CAD build for the part. Positions are in the model's coordinates, mm. A direction names the side the tool comes from. Give positions to 0.01 mm unless a question says otherwise; leave off trailing zeros. Loops run counter-clockwise (first coordinate to the right, second up) from the corner with the lowest first, then second, coordinate; pieces in that order, holes last.
Item 1: Saw through at D-D on y = 0.5. Give the cut face in (x, z).
Item 2: Saw through at B-B on z = 2. Give the cut face in (x, y), plus the area to 3 significant figures.
Item 3: Which spindle directions (+Z, -Z, +X, -X, +Y, -Y) get a long thin tool onto all of the face, cutting with end or side? Do faces 4 (the flat face through (12, -9.083, 5)), 5 (the flat face through (-12.679, -7, 2)), 6 (the flat face through (-13.1, -5, 10)), 7 (the flat face through (-12.679, -7, 17)), 8 (the flat face through (-9, -6, 10)). Say none if no direction does.
Item 4: Saw through at C-C on x = 23.5. Give the cut face in (y, z), plus the area to 3 significant figures.
Item 5: Drop flat-ended pins along their axis: P1, Ø2.5, axis at y = -4.5, z = 6.5, coming from the -X side; P2, Ø12, axis at x = -28.5, z = 15.5, coming from the +Y side; P3, Ø1.5, axis at y = 5.5, z = 2, coming from the +X side. Give the stop position or say it passes through.
Item 6: Probe probe 1 along Y at (x, z) = (-14, 11); probe 2 along Y at (x, z) = (-4, 19); probe 3 along Y at (x, z) = (3, 10.25). List the from-to ranges inside material, lowest first.
Item 7: Mould opens along Y. For faces 1 (the flat face through (20, 1.35, 10.14)), 2 (the flat face through (-10.1, 7, 10)), 3 (the flat face through (-26, -11.5, 10)) say: released by +Y, released by -Y, zero draft, split by the parting line, or undercut.
Item 8: Saw through at A-A on y = -4.75. Give the cut face in (x, z), plus the area to 3 significant figures.
from build123d import *

# Parameters (mm, degrees)
EXTRUDE_1_DEPTH          = 20
CUT_EXTRUDE_1_DEPTH      = 49.817301935
CUT_EXTRUDE_1_DEPTH_BACK = 49.817301935
CUT_EXTRUDE_2_DEPTH      = 50.88447801
CUT_EXTRUDE_2_DEPTH_BACK = 50.88447801
SKETCH_3_W               = 26.81134726
SKETCH_3_H               = 5
CUT_EXTRUDE_3_DEPTH      = 50.88447801
CUT_EXTRUDE_3_DEPTH_BACK = 50.88447801
CUT_EXTRUDE_4_DEPTH      = 50.88447801
CUT_EXTRUDE_4_DEPTH_BACK = 50.88447801
SKETCH_5_R               = 1.55


with BuildPart() as part:
    # 草图1 → 凸台-拉伸1 (new body)
    with BuildSketch(Plane.XY):
        Polygon((-13.100304314, 11.5), (39.490013248, 11.5), (39.490013248, -9.083192704), (1.044300056, -9.083192704), (-7.416317872, -10.795276425), (-10.024002967, -11.323036202), (-12.678665988, -11.5), (-39.490013248, -11.5), (-39.490013248, -7.536083067), (-13.100304314, -7.5), (-13.100304314, -3), (-10.100304314, -3), (-10.100304314, -6), (-7.100304314, -6), (-7.100304314, -2.65), (-3.000304314, -2.65), (-3.000304314, 5.15), (-7.100304314, 5.15), (-7.100304314, 8.5), (-10.100304314, 8.5), (-10.100304314, 5.5), (-13.100304314, 5.5), align=None)
    extrude(amount=EXTRUDE_1_DEPTH)

    # 草图2 → 切除-拉伸1 (cut, two sides: drawn at the far end of the back side and taken through both)
    with BuildSketch(Plane.XZ.offset(9.083192704).offset(-CUT_EXTRUDE_1_DEPTH_BACK)):
        Polygon((1.044300056, 20), (39.490013248, 0), (39.490013248, 20), align=None)
    extrude(amount=CUT_EXTRUDE_1_DEPTH + CUT_EXTRUDE_1_DEPTH_BACK, mode=Mode.SUBTRACT)

    # 草图3 → 切除-拉伸2 (cut, two sides: drawn at the far end of the back side and taken through both)
    with BuildSketch(Plane.XZ.offset(11.5).offset(-CUT_EXTRUDE_2_DEPTH_BACK)):
        with Locations((-26.084339618, 17.5)):
            Rectangle(SKETCH_3_W, SKETCH_3_H)
        with Locations((-26.084339618, 2.5)):
            Rectangle(SKETCH_3_W, SKETCH_3_H)
    extrude(amount=CUT_EXTRUDE_2_DEPTH + CUT_EXTRUDE_2_DEPTH_BACK, mode=Mode.SUBTRACT)

    # 草图4 → 切除-拉伸3 (cut, two sides: drawn at the far end of the back side and taken through both)
    with BuildSketch(Plane.XZ.offset(11.5).offset(-CUT_EXTRUDE_3_DEPTH_BACK)):
        with BuildLine():
            ThreePointArc((-39.490013248, 10), (-38.025547154, 13.535533906), (-34.490013248, 15))
            Line((-34.490013248, 15), (-39.490013248, 15))
            Line((-39.490013248, 15), (-39.490013248, 10))
        make_face()
        with BuildLine():
            ThreePointArc((-34.490013248, 5), (-38.025547154, 6.464466094), (-39.490013248, 10))
            Line((-39.490013248, 10), (-39.490013248, 5))
            Line((-39.490013248, 5), (-34.490013248, 5))
        make_face()
    extrude(amount=CUT_EXTRUDE_3_DEPTH + CUT_EXTRUDE_3_DEPTH_BACK, mode=Mode.SUBTRACT)

    # 草图5 → 切除-拉伸4 (cut, two sides: drawn at the far end of the back side and taken through both)
    with BuildSketch(Plane.XZ.offset(11.5).offset(-CUT_EXTRUDE_4_DEPTH_BACK)):
        with Locations(Location((-34.490013248, 10, 0), (0, 0, 180))):
            Circle(SKETCH_5_R)
    extrude(amount=CUT_EXTRUDE_4_DEPTH + CUT_EXTRUDE_4_DEPTH_BACK, mode=Mode.SUBTRACT)


solid = part.part
Results below:
1. outline: (-3, 0) - (39.49, 0) - (1.04, 20) - (-3, 20) - close
2. outline: (-12.68, -11.5) - (-10.02, -11.32) - (-7.42, -10.8) - (1.04, -9.08) - (35.65, -9.08) - (35.65, 11.5) - (-12.68, 11.5) - (-12.68, 5.5) - (-10.1, 5.5) - (-10.1, 8.5) - (-7.1, 8.5) - (-7.1, 5.15) - (-3, 5.15) - (-3, -2.65) - (-7.1, -2.65) - (-7.1, -6) - (-10.1, -6) - (-10.1, -3) - (-12.68, -3) - close
2. area: 916 mm2
3. face 4: +Z, -Z, +X, -Y
3. face 5: -Z, -X, +Y, -Y
3. face 6: +Z, -Z, -X, +Y
3. face 7: +Z, -X, +Y, -Y
3. face 8: +Z, -Z
4. outline: (-9.08, 0) - (11.5, 0) - (11.5, 8.32) - (-9.08, 8.32) - close
4. area: 171 mm2
5. P1: stops at x = -13.1
5. P2: stops at y = -7.51
5. P3: stops at x = 37.09
6. probe 1: y = -11.5 to -7.5
6. probe 2: y = -10.1 to -2.65, 5.15 to 11.5
6. probe 3: y = -9.08 to 11.5
7. face 1: zero draft
7. face 2: undercut
7. face 3: released by -Y
8. outline: (-13.1, 5) - (-12.68, 5) - (-12.68, 0) - (-10.1, 0) - (-10.1, 20) - (-12.68, 20) - (-12.68, 15) - (-13.1, 15) - close; (-7.1, 0) - (39.49, 0) - (1.04, 20) - (-7.1, 20) - close
8. area: 603 mm2
